Build history of the part. All positions in model axes, mm. Face numbers are marked on the shaded views. A direction names the side the tool comes from. Coordinates: 2 decimals unless noted, no trailing zeros. Write each loop counter-clockwise with the first axis right and the second up, starting at its lowest first coordinate (ties: lowest second). Pieces come first, ordered by that corner, then holes.
```python
from build123d import *

# Parameters (mm, degrees)
BOSS_EXTRUDE1_DEPTH = 20
SKETCH2_W           = 5
SKETCH2_H           = 72.5
BOSS_EXTRUDE2_DEPTH = 60
SKETCH3_R           = 15
CUT_EXTRUDE1_DEPTH  = 100
SKETCH4_R           = 1.25
CUT_EXTRUDE2_DEPTH  = 100
SKETCH7_W           = 77.5
SKETCH7_H           = 5
BOSS_EXTRUDE6_DEPTH = 60
FILLET3_R           = 5
SKETCH8_W           = 25
SKETCH8_H           = 120
SKETCH8_H_2         = 25
SKETCH8_W_2         = 120
CUT_EXTRUDE3_DEPTH  = 100
SKETCH9_R           = 1.65
CUT_EXTRUDE4_DEPTH  = 100
SKETCH10_W          = 42.5
SKETCH10_H          = 42.5
SKETCH10_W_2        = 77.5
SKETCH10_H_2        = 77.5
CUT_EXTRUDE5_DEPTH  = 15
FILLET4_R           = 10
SKETCH11_W          = 20
SKETCH11_H          = 5
CUT_EXTRUDE6_DEPTH  = 6
FILLET5_R           = 5


with BuildPart() as part:
    # Sketch1 → Boss-Extrude1 (new body)
    with BuildSketch(Plane(origin=(0, 0, 0), x_dir=(1, 0, 0), z_dir=(0, 1, 0))):
        Polygon((72.5, 72.5), (0, 72.5), (0, 0), (-72.5, 0), (-72.5, -72.5), (72.5, -72.5), align=None)
    extrude(amount=BOSS_EXTRUDE1_DEPTH)

    # Sketch2 → Boss-Extrude2 (add)
    with BuildSketch(Plane(origin=(0, 20, 0), x_dir=(1, 0, 0), z_dir=(0, 1, 0))):
        with Locations((2.5, 36.25)):
            Rectangle(SKETCH2_W, SKETCH2_H)
    extrude(amount=BOSS_EXTRUDE2_DEPTH)

    # Sketch3 → Cut-Extrude1 (cut)
    with BuildSketch(Plane.ZY):
        with Locations((-47.5, 58.85)):
            Circle(SKETCH3_R)
    cut_extrude1 = extrude(amount=-CUT_EXTRUDE1_DEPTH, mode=Mode.SUBTRACT)

    # Sketch4 → Cut-Extrude2 (cut)
    with BuildSketch(Plane.ZY):
        with Locations((-32, 74.35)):
            Circle(SKETCH4_R)
        with Locations((-63, 74.35)):
            Circle(SKETCH4_R)
        with Locations((-63, 43.35)):
            Circle(SKETCH4_R)
        with Locations((-32, 43.35)):
            Circle(SKETCH4_R)
    cut_extrude2 = extrude(amount=-CUT_EXTRUDE2_DEPTH, mode=Mode.SUBTRACT)

    # Sketch7 → Boss-Extrude6 (add)
    with BuildSketch(Plane(origin=(0, 20, 0), x_dir=(1, 0, 0), z_dir=(0, 1, 0))):
        with Locations((-33.75, -2.5)):
            Rectangle(SKETCH7_W, SKETCH7_H)
    extrude(amount=BOSS_EXTRUDE6_DEPTH)

    # Mirror5: Cut-Extrude1, Cut-Extrude2 across plane
    add(cut_extrude1.mirror(Plane(origin=(0, 0, 0), x_dir=(0.7071067811865476, 0, 0.7071067811865475), z_dir=(-0.7071067811865475, 0, 0.7071067811865476))), mode=Mode.SUBTRACT)
    add(cut_extrude2.mirror(Plane(origin=(0, 0, 0), x_dir=(0.7071067811865476, 0, 0.7071067811865475), z_dir=(-0.7071067811865475, 0, 0.7071067811865476))), mode=Mode.SUBTRACT)

    # Fillet3
    fillet3_edges = [part.edges().sort_by_distance(p)[0] for p in [
        (0, 40, 0),
    ]]
    fillet(fillet3_edges, radius=FILLET3_R)

    # Sketch8 → Cut-Extrude3 (cut)
    with BuildSketch(Plane(origin=(0, 20, 0), x_dir=(1, 0, 0), z_dir=(0, 1, 0))):
        with Locations((60, 12.5)):
            Rectangle(SKETCH8_W, SKETCH8_H)
        with Locations((60, -60)):
            Rectangle(SKETCH8_W, SKETCH8_H_2)
        with Locations((-12.5, -60)):
            Rectangle(SKETCH8_W_2, SKETCH8_H_2)
    extrude(amount=-CUT_EXTRUDE3_DEPTH, mode=Mode.SUBTRACT)

    # Sketch9 → Cut-Extrude4 (cut)
    with BuildSketch(Plane(origin=(0, 20, 0), x_dir=(1, 0, 0), z_dir=(0, 1, 0))):
        with Locations(Location((42.5, 67.5, 0), (0, 0, 270))):
            Circle(SKETCH9_R)
        with Locations(Location((42.5, -42.5, 0), (0, 0, 270))):
            Circle(SKETCH9_R)
        with Locations(Location((-67.5, -42.5, 0), (0, 0, 270))):
            Circle(SKETCH9_R)
    extrude(amount=-CUT_EXTRUDE4_DEPTH, mode=Mode.SUBTRACT)

    # Sketch10 → Cut-Extrude5 (cut)
    with BuildSketch(Plane(origin=(0, 20, 0), x_dir=(1, 0, 0), z_dir=(0, 1, 0))):
        with Locations((26.25, -26.25)):
            Rectangle(SKETCH10_W, SKETCH10_H)
        with Locations((-33.75, -26.25)):
            Rectangle(SKETCH10_W_2, SKETCH10_H)
        with Locations((26.25, 33.75)):
            Rectangle(SKETCH10_W, SKETCH10_H_2)
    extrude(amount=-CUT_EXTRUDE5_DEPTH, mode=Mode.SUBTRACT)

    # Fillet4
    fillet4_edges = [part.edges().sort_by_distance(p)[0] for p in [
        (5, 5, -33.75),
        (-33.75, 5, 5),
        (5, 42.5, 5),
    ]]
    fillet(fillet4_edges, radius=FILLET4_R)

    # Sketch11 → Cut-Extrude6 (cut)
    with BuildSketch(Plane.XY.offset(5)):
        with Locations((-47.5, 28.85)):
            Rectangle(SKETCH11_W, SKETCH11_H)
    extrude(amount=-CUT_EXTRUDE6_DEPTH, mode=Mode.SUBTRACT)

    # Fillet5
    # the kernel refuses this fillet: 5 mm, written as the material it adds along each edge
    with BuildSketch(Plane(origin=(-57.5, 26.35, 5), x_dir=(1, 0, 0), z_dir=(0, 0, -1))) as fillet5_piece_1:
        with BuildLine():
            CenterArc((FILLET5_R, -FILLET5_R), FILLET5_R, 90, 90)
            Line((0, -FILLET5_R), (0, 0))
            Line((0, 0), (FILLET5_R, 0))
        make_face()
    extrude(amount=5)
    with BuildSketch(Plane(origin=(-57.5, 31.35, 5), x_dir=(1, 0, 0), z_dir=(0, 0, -1)), Plane(origin=(-37.5, 31.35, 5), x_dir=(0, -1, 0), z_dir=(0, 0, -1)), Plane(origin=(-37.5, 26.35, 5), x_dir=(-1, 0, 0), z_dir=(0, 0, -1))) as fillet5_piece_2:
        with BuildLine():
            CenterArc((FILLET5_R, FILLET5_R), FILLET5_R, 180, 90)
            Line((0, FILLET5_R), (0, 0))
            Line((0, 0), (FILLET5_R, 0))
        make_face()
    extrude(amount=5)


solid = part.part
```
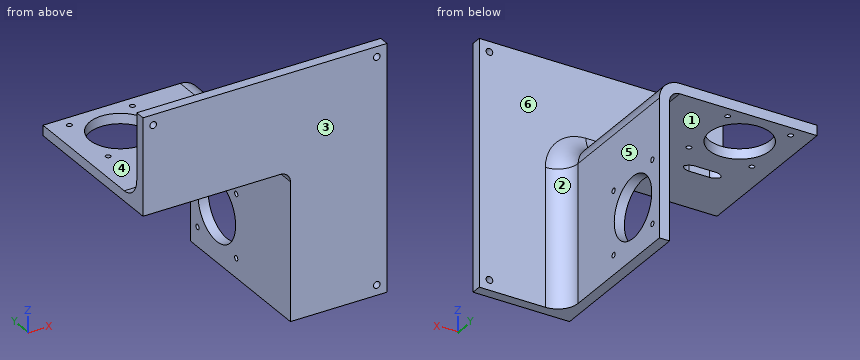
1. Saw through at B-B on z = -67.5. List the corners of the cut face in (x, y).
Computed values:
outline: (0, 0) - (40.85, 0) - (40.85, 5) - (15, 5) arc R10 cw to (5, 15) - (5, 80) - (0, 80) - close; (44.15, 0) - (47.5, 0) - (47.5, 5) - (44.15, 5) - close
2. Saw through at D-D on y = 62.5. List the corners of the cut face in (x, z).
Computed values:
outline: (-72.5, 0) - (-62.05, 0) - (-62.05, 5) - (-72.5, 5) - close; (-32.95, 0) - (-5, 0) arc R5 cw to (0, -5) - (0, -32.95) - (5, -32.95) - (5, -5) arc R10 ccw to (-5, 5) - (-32.95, 5) - close; (0, -72.5) - (5, -72.5) - (5, -62.05) - (0, -62.05) - close
3. Saw through at A-A on x = 42.5. List the corners of the cut face in (y, z), plus the area to 3 significant figures.
Computed values:
outline: (0, -72.5) - (5, -72.5) - (5, -69.15) - (0, -69.15) - close; (0, -65.85) - (5, -65.85) - (5, 40.85) - (0, 40.85) - close; (0, 44.15) - (5, 44.15) - (5, 47.5) - (0, 47.5) - close
area: 567 mm2
4. Mould opens along Y. For the marked faces 1, 2 and 3 say: +Y half, -Y half, draft (parallel to the pull), parting line (faces both ways), or undercut.
Computed values:
face 1: draft
face 2: +Y half
face 3: -Y half
5. Probe line 1 along Y through (x, z) = (-32, 2.45); line 2 along X through (y, z) = (1.45, 42.5); line 3 along Z through (x, y) = (1, 74). List the from-to ranges inside material, lowest first.
Computed values:
line 1: y = 0 to 42.1, 44.6 to 73.1, 75.6 to 80
line 2: x = -72.5 to -69.15, -65.85 to 40.85, 44.15 to 47.5
line 3: z = -72.5 to -64.2, -61.8 to -33.2, -30.8 to 3
6. 3-axis set-ups, long thin cutter, end or side, ignore diameter. For the marked faces 4, 5 and 6: which of +Z, -Z, +X, -X, +Y, -Y reach the whole face in a straight line?
Computed values:
face 4: +Z, +X, -X, +Y
face 5: +Z, -Z, +X, +Y
face 6: +Z, +X, +Y
7. Saw through at C-C on z = 42.5. List the corners of the cut face in (x, y).
Computed values:
outline: (-72.5, 0) - (-69.15, 0) - (-69.15, 5) - (-72.5, 5) - close; (-65.85, 0) - (40.85, 0) - (40.85, 5) - (-65.85, 5) - close; (44.15, 0) - (47.5, 0) - (47.5, 5) - (44.15, 5) - close
8. Flat gauge pins, fed straight in: pin 1 (4 mm diameter, centred on x = -46, z = 2.5, fed in from -Y); pin 2 (3 mm diameter, centred on y = 43.35, z = -32, fed in from -X); pin 3 (8 mm diameter, centred on x = -38.5, y = 14.5, fed in from -Z); pin 4 (3 mm diameter, centred on x = -63, y = 74.35, fed in from +Z). Where does each tip first touch, or does it go through?
Computed values:
pin 1: stops at y = 0
pin 2: stops at x = 0
pin 3: stops at z = 0
pin 4: stops at z = 5
